from build123d import *

# Parameters (mm, degrees)
SKETCH1_W           = 152.4
SKETCH1_H           = 165.1
BOSS_EXTRUDE1_DEPTH = 3.175
CUT_EXTRUDE1_DEPTH  = 4.175
SKETCH3_R           = 3.96875
CUT_EXTRUDE2_DEPTH  = 4.175


with BuildPart() as part:
    # Sketch1 → Boss-Extrude1 (new body)
    with BuildSketch(Plane(origin=(0, 0, 0), x_dir=(0, 0, -1), z_dir=(1, 0, 0))):
        with Locations((76.2, 0)):
            Rectangle(SKETCH1_W, SKETCH1_H)
    extrude(amount=BOSS_EXTRUDE1_DEPTH)

    # Sketch2 → Cut-Extrude1 (cut, through all)
    with BuildSketch(Plane.ZY):
        with BuildLine():
            Line((-107.95, 25.4), (-107.95, -25.4))
            ThreePointArc((-107.95, -25.4), (-106.090128061, -29.890128061), (-101.6, -31.75))
            Line((-101.6, -31.75), (-50.8, -31.75))
            ThreePointArc((-50.8, -31.75), (-46.309871939, -29.890128061), (-44.45, -25.4))
            Line((-44.45, -25.4), (-44.45, 25.4))
            ThreePointArc((-44.45, 25.4), (-46.309871939, 29.890128061), (-50.8, 31.75))
            Line((-50.8, 31.75), (-101.6, 31.75))
            ThreePointArc((-101.6, 31.75), (-106.090128061, 29.890128061), (-107.95, 25.4))
        make_face()
    extrude(amount=-CUT_EXTRUDE1_DEPTH, mode=Mode.SUBTRACT)

    # Sketch3 → Cut-Extrude2 (cut, through all)
    with BuildSketch(Plane.ZY):
        with Locations((-60.325, 69.85)):
            Circle(SKETCH3_R)
        with Locations((-92.075, 69.85)):
            Circle(SKETCH3_R)
        with Locations((-92.075, -69.85)):
            Circle(SKETCH3_R)
        with Locations((-60.325, -69.85)):
            Circle(SKETCH3_R)
    extrude(amount=-CUT_EXTRUDE2_DEPTH, mode=Mode.SUBTRACT)


solid = part.part
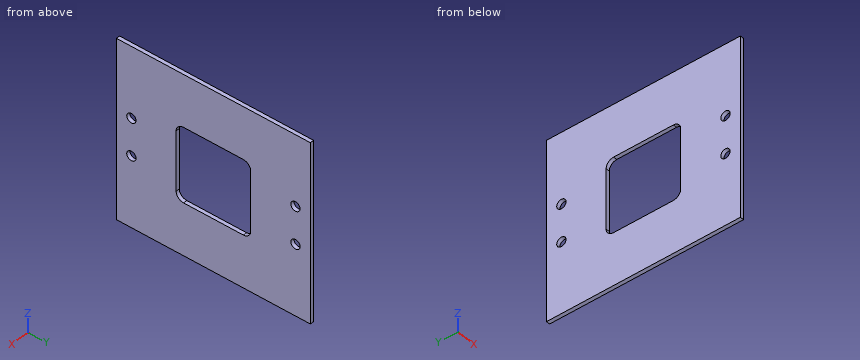
Geometry: final body of the model. Coordinates: model frame, mm. Round coordinates to 2 decimals unless told otherwise and drop trailing zeros. Write each loop counter-clockwise with the first axis right and the second up, starting at its lowest first coordinate (ties: lowest second). Pieces come first, ordered by that corner, then holes. Notation, with made-up numbers: M 40,5 L 98,5 A21 cw 98,40 Z; hole C -6,1 d2. An arc over 180 degrees is marked long. Write item = value, one per line.
Item 1: Material intervals for line 1 along Y through (x, z) = (2.5, -91.5); line 2 along Z through (x, y) = (0.65, -67); line 3 along Y through (x, z) = (2.85, -86.5), sorted ascending. Write a range as [from, to].
Findings:
line_1 = [-82.55, -73.78], [-65.92, -31.75], [31.75, 65.92], [73.78, 82.55]
line_2 = [-152.4, -94.84], [-89.31, -63.09], [-57.56, 0]
line_3 = [-82.55, -31.75], [31.75, 82.55]
Item 2: Section query C-C on y = -69.85. Return loops of the section in (x, z) (3 decimals).
Findings:
outline = M 0,-152.4 L 3.175,-152.4 L 3.175,-96.044 L 0,-96.044 Z; M 0,-88.106 L 3.175,-88.106 L 3.175,-64.294 L 0,-64.294 Z; M 0,-56.356 L 3.175,-56.356 L 3.175,0 L 0,0 Z
Item 3: Section query B-B on x = 0.7. State how many separate pieces and enclosed holes the cut face has, then the cut area to 3 significant figures.
Findings:
separate_pieces = 1
enclosed_holes = 5
area = 21,000 mm^2
Item 4: Section query A-A on y = 0. Return loops of the section in (x, z) (3 decimals), then the cut area to 3 significant figures.
Findings:
outline = M 0,-152.4 L 3.175,-152.4 L 3.175,-107.95 L 0,-107.95 Z; M 0,-44.45 L 3.175,-44.45 L 3.175,0 L 0,0 Z
area = 282 mm^2
